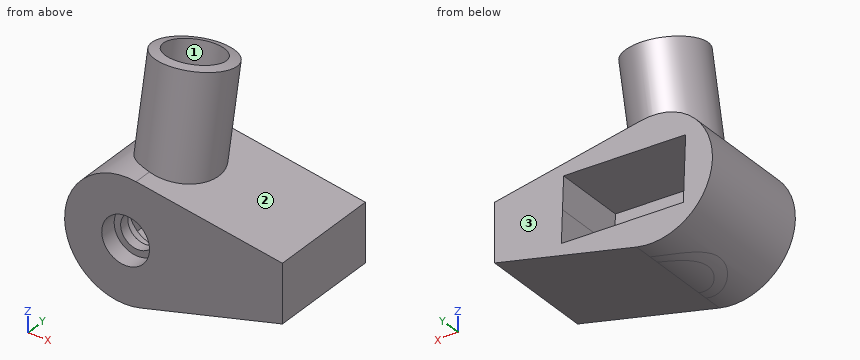
```python
from build123d import *

# Parameters (mm, degrees)
CROQUIS1_R              = 21
SALIENTE_EXTRUIR1_DEPTH = 40
SALIENTE_EXTRUIR2_DEPTH = 40
SALIENTE_EXTRUIR3_REACH = 77.493
CROQUIS3_R              = 13.5
CROQUIS3_R_2            = 10
CROQUIS7_R              = 8.227269221
CROQUIS7_R_2            = 6
CORTAR_EXTRUIR6_DEPTH   = 6
CROQUIS8_R              = 6
CORTAR_EXTRUIR7_DEPTH   = 72.223648425
CORTAR_EXTRUIR8_START   = -25
CORTAR_EXTRUIR8_DEPTH   = 25
CROQUIS12_R             = 9.55
CORTAR_EXTRUIR9_DEPTH   = 5.5
CORTAR_EXTRUIR10_DEPTH  = 86.45696425


with BuildPart() as part:
    # Croquis1 → Saliente-Extruir1 (new body)
    with BuildSketch(Plane(origin=(0, 0, 0), x_dir=(1, 0, 0), z_dir=(0, 1, 0))):
        with Locations(Location((0, 0, 0), (0, 0, 270))):
            Circle(CROQUIS1_R)
    extrude(amount=SALIENTE_EXTRUIR1_DEPTH)

    # Croquis2 → Saliente-Extruir2 (add)
    with BuildSketch(Plane(origin=(0, 0, 0), x_dir=(1, 0, 0), z_dir=(0, 1, 0))):
        with BuildLine():
            Line((53.975127576, 8.110971331), (53.975127576, -11.889028669))
            Line((53.975127576, -11.889028669), (3.613793412, -20.686722727))
            ThreePointArc((3.613793412, -20.686722727), (20.98607707, -0.764571273), (5.109545014, 20.368911354))
            Line((5.109545014, 20.368911354), (53.975127576, 8.110971331))
        make_face()
    extrude(amount=SALIENTE_EXTRUIR2_DEPTH)

    # Croquis3 → Saliente-Extruir3 (add, up to next)
    with BuildSketch(Plane(origin=(5.109545014, 0, -20.368911354), x_dir=(-0.9699481597219111, 0, -0.24331166731597212), z_dir=(0.2433116673159721, 0, -0.969948159721911)), mode=Mode.PRIVATE) as saliente_extruir3_sk1:
        with Locations((0, 20)):
            Circle(CROQUIS3_R)
        with Locations((0, 20)):
            Circle(CROQUIS3_R_2, mode=Mode.SUBTRACT)
    saliente_extruir3_tool1 = extrude(saliente_extruir3_sk1.sketch, amount=-SALIENTE_EXTRUIR3_REACH, mode=Mode.PRIVATE) - part.part
    add(saliente_extruir3_tool1.solids().sort_by_distance((17.833482, 20, -17.177109))[0])

    # Croquis7 → Cortar-Extruir6 (cut)
    with BuildSketch(Plane.XZ):
        with Locations(Location((0, 0, 0), (0, 0, 270))):
            Circle(CROQUIS7_R)
        with Locations(Location((0, 0, 0), (0, 0, 270))):
            Circle(CROQUIS7_R_2, mode=Mode.SUBTRACT)
    extrude(amount=-CORTAR_EXTRUIR6_DEPTH, mode=Mode.SUBTRACT)

    # Croquis8 → Cortar-Extruir7 (cut, through all)
    with BuildSketch(Plane.XZ):
        with Locations(Location((0, 0, 0), (0, 0, 270))):
            Circle(CROQUIS8_R)
    extrude(amount=-CORTAR_EXTRUIR7_DEPTH, mode=Mode.SUBTRACT)

    # Croquis10 → Cortar-Extruir8 (cut)
    with BuildSketch(Plane(origin=(0, 40, 0), x_dir=(1, 0, 0), z_dir=(0, 1, 0)).offset(CORTAR_EXTRUIR8_START)):
        with BuildLine():
            Line((-5.995438853, 0.23390802), (-11.37823559, 0.424457107))
            Line((-11.37823559, 0.424457107), (-11.767631672, -10.575542893))
            Line((-11.767631672, -10.575542893), (30.232368328, -12.062327932))
            Line((30.232368328, -12.062327932), (30.62176441, -1.062327932))
            Line((30.62176441, -1.062327932), (5.996971268, -0.190619027))
            ThreePointArc((5.996971268, -0.190619027), (-0.212264906, -5.996244125), (-5.995438853, 0.23390802))
        make_face()
        with BuildLine():
            Line((-10.988839509, 11.424457107), (-11.37823559, 0.424457107))
            Line((-11.37823559, 0.424457107), (-5.995438853, 0.23390802))
            ThreePointArc((-5.995438853, 0.23390802), (0.116976243, 5.998859605), (6, 0))
            ThreePointArc((6, 0), (5.999242769, -0.095321543), (5.996971268, -0.190619027))
            Line((5.996971268, -0.190619027), (30.62176441, -1.062327932))
            Line((30.62176441, -1.062327932), (31.011160491, 9.937672068))
            Line((31.011160491, 9.937672068), (-10.988839509, 11.424457107))
        make_face()
    extrude(amount=CORTAR_EXTRUIR8_DEPTH, mode=Mode.SUBTRACT)

    # Croquis12 → Cortar-Extruir9 (cut)
    with BuildSketch(Plane(origin=(0, 15, 0), x_dir=(1, 0, 0), z_dir=(0, 1, 0))):
        with Locations(Location((0, 0, 0), (0, 0, 270))):
            Circle(CROQUIS12_R)
    extrude(amount=-CORTAR_EXTRUIR9_DEPTH, mode=Mode.SUBTRACT)

    # Croquis4 → Revolución3 (revolve)
    with BuildSketch(Plane(origin=(5.1, 0, 0), x_dir=(0, 0, -1), z_dir=(1, 0, 0)), mode=Mode.PRIVATE) as revoluci_n3_sk:
        Polygon((-24.61645883, 10.663524112), (-17.776790486, 9.208275528), (-17.776790486, 5.708275528), (-52.81645883, 13.163524112), (-52.81645883, 16.663524112), align=None)
    revolve(revoluci_n3_sk.sketch.rotate(Axis((5.1, 20.663524112, 24.61645883), (0, 0.20810764446485971, 0.9781059289848353)), 180), axis=Axis((5.1, 20.663524112, 24.61645883), (0, 0.20810764446485971, 0.9781059289848353)))

    # Croquis17 → Cortar-Extruir10 (cut, through all)
    with BuildSketch(Plane(origin=(0, 40, 0), x_dir=(1, 0, 0), z_dir=(0, 1, 0))):
        with BuildLine():
            Line((5.109545014, 20.368911354), (5.109545014, 31.680559043))
            Line((5.109545014, 31.680559043), (-13.688349404, 31.680559043))
            Line((-13.688349404, 31.680559043), (-13.688349404, 15.925736736))
            ThreePointArc((-13.688349404, 15.925736736), (-4.830571536, 20.436868122), (5.109545014, 20.368911354))
        make_face()
    extrude(amount=-CORTAR_EXTRUIR10_DEPTH, mode=Mode.SUBTRACT)


solid = part.part
```
Can you work these out from the model? Positions are in its coordinate system, mm. Face numbers are marked on the shaded views. Coordinates: 2 decimals unless noted, no trailing zeros. Loops run counter-clockwise (first coordinate to the right, second up) from the corner with the lowest first, then second, coordinate; pieces in that order, holes last.
Item 1: Suppose I cut it at A-A (y = 34.5). State how many separate pieces and enclosed holes the cut face has, then the cut area to 3 significant figures.
Answers below:
separate pieces: 2
enclosed holes: 1
area: 1,740 mm2
Item 2: Suppose I cut it at B-B (z = -3). Please give me the cut outline in (x, y).
Answers below:
outline: (-20.78, 0) - (-7.66, 0) - (-7.66, 6) - (-5.2, 6) - (-5.2, 9.5) - (-9.07, 9.5) - (-9.07, 15) - (-11.29, 15) - (-11.29, 40) - (-20.78, 40) - close; (5.2, 6) - (7.66, 6) - (7.66, 0) - (53.98, 0) - (53.98, 40) - (30.77, 40) - (30.77, 15) - (9.07, 15) - (9.07, 9.5) - (5.2, 9.5) - close
Item 3: If we mould it in two halves opening along X, with no side actions, what happens to the marked faces 1, 2 and 3? For each: released by +X, released by -X, zero draft, split by the parting line, or undercut.
Answers below:
face 1: undercut
face 2: released by +X
face 3: zero draft
Item 4: Please list where these lines run through material, in increasing order: L1, parallel to X at y = 2, z = 0; L2, parallel to X at y = 8.7, z = 0; L3, parallel to Y at x = 14, z = 29.5.
Answers below:
L1: x = -21 to -8.23, 8.23 to 53.98
L2: x = -21 to -6, 6 to 53.98
L3: y = 11.73 to 17.55, 25.85 to 31.68
Item 5: I'm going to push flat-ended pins straight in: pin 1 (8 mm diameter, centred on x = 35, y = 21, fed in from +Z); pin 2 (13 mm diameter, centred on x = 1, z = 3, fed in from -Y); pin 3 (12 mm diameter, centred on x = -9.5, y = 33, fed in from +Z); pin 4 (11.5 mm diameter, centred on x = 15, z = -2, fed in from +Y). Where does each tip first touch, or does it pass through?
Answers below:
pin 1: stops at z = 15.9
pin 2: stops at y = 0
pin 3: stops at z = 50.06
pin 4: stops at y = 15
Item 6: Suppose I cut it at C-C (y = 4). Please give me the cut outline in (x, z).
Answers below:
outline: (3.61, 20.69) arc R21 ccw (long way) to (5.11, -20.37) - (53.98, -8.11) - (53.98, 11.89) - close; hole circle Ø16.45 at (0, 0)
Item 7: Suppose I cut it at D-D (z = 16.5). Please give me the cut outline in (x, y), then the cut area to 3 significant figures.
Answers below:
outline: (-12.99, 0) - (27.58, 0) - (27.58, 40) - (-12.99, 40) - close
area: 1,620 mm2
